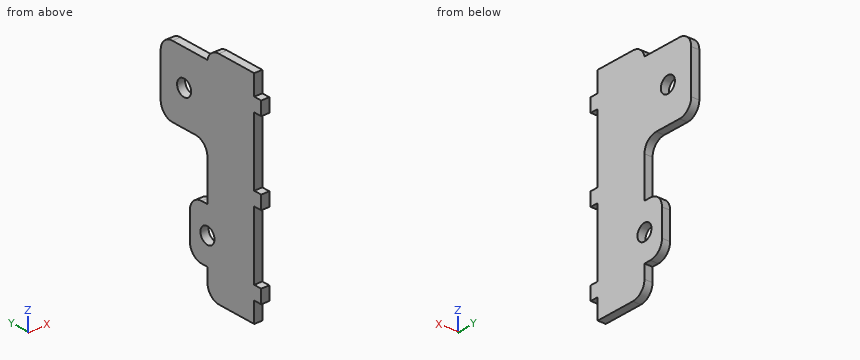
```python
from build123d import *

# Parameters (mm, degrees)
SKETCH1_W           = 80
SKETCH1_H           = 40
BOSS_EXTRUDE1_DEPTH = 3
SKETCH2_R           = 3
SKETCH2_W           = 4
SKETCH2_H           = 20
CUT_EXTRUDE1_DEPTH  = 65.101482042
FILLET2_R           = 5
SKETCH3_W           = 3
SKETCH3_H           = 5
BOSS_EXTRUDE2_DEPTH = 3
LPATTERN1_COUNT     = 3
LPATTERN1_PITCH     = 30


with BuildPart() as part:
    # Sketch1 → Boss-Extrude1 (new body)
    with BuildSketch(Plane(origin=(0, 0, 0), x_dir=(0, 0, -1), z_dir=(1, 0, 0))):
        with Locations((10, 20)):
            Rectangle(SKETCH1_W, SKETCH1_H)
    extrude(amount=BOSS_EXTRUDE1_DEPTH)

    # Sketch2 → Cut-Extrude1 (cut, through all)
    with BuildSketch(Plane(origin=(3, 0, 0), x_dir=(0, 0, -1), z_dir=(1, 0, 0))):
        with Locations((30, 20)):
            Circle(SKETCH2_R)
        with Locations((-13, 30)):
            Circle(SKETCH2_R)
        Polygon((0, 40), (50, 40), (50, 27.5), (50, 20), (40, 20), (40, 27.5), (20, 27.5), (20, 20), (0, 20), (0, 27.5), align=None)
        with Locations((-28, 30)):
            Rectangle(SKETCH2_W, SKETCH2_H)
    extrude(amount=-CUT_EXTRUDE1_DEPTH, mode=Mode.SUBTRACT)

    # Fillet2
    # the kernel refuses this fillet: 5 mm, written as the material it adds along each edge
    with BuildSketch(Plane(origin=(3, 20, 0), x_dir=(0, 0, -1), z_dir=(-1, 0, 0))) as fillet2_piece_1:
        with BuildLine():
            CenterArc((FILLET2_R, -FILLET2_R), FILLET2_R, 90, 90)
            Line((0, -FILLET2_R), (0, 0))
            Line((0, 0), (FILLET2_R, 0))
        make_face()
    extrude(amount=3)
    # the kernel refuses this fillet: 5 mm, written as the material it takes off along each edge
    with BuildSketch(Plane(origin=(15.5, 40, 26), x_dir=(0, 0, -1), z_dir=(-1, 0, 0)), Plane(origin=(15.5, 27.5, -40), x_dir=(0, -1, 0), z_dir=(-1, 0, 0)), Plane(origin=(15.5, 27.5, -20), x_dir=(0, 0, -1), z_dir=(-1, 0, 0)), Plane(origin=(15.5, 40, 0), x_dir=(0, -1, 0), z_dir=(-1, 0, 0)), Plane(origin=(15.5, 20, -50), x_dir=(0, -1, 0), z_dir=(-1, 0, 0))) as fillet2_2_piece_1:
        with BuildLine():
            CenterArc((FILLET2_R, FILLET2_R), FILLET2_R, 180, 90)
            Line((0, FILLET2_R), (0, 0))
            Line((0, 0), (FILLET2_R, 0))
        make_face()
    extrude(amount=28, mode=Mode.SUBTRACT)
    with BuildSketch(Plane(origin=(15.247448714, 20, 30), x_dir=(0, -1, 0), z_dir=(-1, 0, 0))) as fillet2_2_piece_2:
        with BuildLine():
            CenterArc((4.898979486, -5), FILLET2_R, 90, 78.463040967)
            Line((0, -4), (0, 0))
            Line((0, 0), (4.898979486, 0))
        make_face()
    extrude(amount=27.494897428, mode=Mode.SUBTRACT)

    # Sketch3 → Boss-Extrude2 (add)
    with BuildSketch(Plane.XZ):
        with Locations((1.5, -40)):
            Rectangle(SKETCH3_W, SKETCH3_H)
    boss_extrude2 = extrude(amount=BOSS_EXTRUDE2_DEPTH)

    # LPattern1: Boss-Extrude2 ×3
    with Locations(*[(0, 0, i * LPATTERN1_PITCH) for i in range(1, LPATTERN1_COUNT)]):
        add(boss_extrude2)


solid = part.part
```
Could you check a few things on this model? Use its own coordinates, in mm. Round coordinates to 2 decimals unless told otherwise and drop trailing zeros. Order: outer loops, then holes, each group sorted by start corner. A loop starts at its lowest first (then second) coordinate and runs counter-clockwise, first axis right, second up. Notation, with made-up numbers: M 24,0 L 52,0 A10 cw 52,14 Z; hole C 79,-33.5 d5. An arc over 180 degrees is marked long. One line per question, with ' | ' between items. Start each with the question number.
(1) For P1, Ø0.9, axis at x = 1, z = -29.5, coming from the +Y side; P2, Ø1.5, axis at x = 2, y = -1.5, coming from the +Z side; P3, Ø0.9, axis at x = 2, z = -26, coming from the -Y side; P4, Ø10, axis at y = 32, z = -19.5, coming from the +X side, each with a flat end and sliding along its axis, tell me the tip position at first contact or that it passes through.
(2) Suppose I cut it at B-B on x = 1.75. Count the separate pieces of the cut face and the enclosed holes in it, then the cut area to 3 significant figures.
(3) Suppose I cut it at D-D on z = -39. List the corners of the cut face in (x, y) for me.
(4) Please list where these lines run through material, in increasing order: line 1 along Y through (x, z) = (2.35, 13); line 2 along Z through (x, y) = (1.15, -0.5); line 3 along Y through (x, z) = (2.05, -30).
(5) Suppose I cut it at C-C on z = -30. List the corners of the cut face in (x, y) for me, then the cut area to 3 significant figures.
(6) Suppose I cut it at A-A on y = 30. List the corners of the cut face in (x, z) for me.
Geometry results:
1) P1: y = 27.5 | P2: z = 22.5 | P3: y = 0 | P4: through
2) separate pieces: 1 | enclosed holes: 2 | area: 2,230 mm²
3) outline: M 0,-3 L 3,-3 L 3,25.5 L 0,25.5 Z
4) line 1: 0 to 27, 33 to 40 | line 2: -42.5 to -37.5, -12.5 to -7.5, 17.5 to 22.5 | line 3: 0 to 17, 23 to 27.5
5) outline: M 0,0 L 3,0 L 3,17 L 0,17 Z; M 0,23 L 3,23 L 3,27.5 L 0,27.5 Z | area: 64.5 mm²
6) outline: M 0,0 L 3,0 L 3,10 L 0,10 Z; M 0,16 L 3,16 L 3,26 L 0,26 Z
